Geometry: final body of the model. Coordinates: model frame, mm. A direction names the side the tool comes from. Round coordinates to 2 decimals unless told otherwise and drop trailing zeros. Write each loop counter-clockwise with the first axis right and the second up, starting at its lowest first coordinate (ties: lowest second). Pieces come first, ordered by that corner, then holes.
from build123d import *

# Parameters (mm, degrees)
F0_W      = 50.8
F0_H      = 457.2
F1_DEPTH  = 50.8
F2_R      = 4.699
F3_DEPTH  = 50.801
F5_DEPTH  = 50.801
F7_R      = 21.0312
F8_DEPTH  = 12.7
F9_R      = 16.002
F10_DEPTH = 12.7
F11_R     = 16.002
F12_DEPTH = 12.7
F13_R     = 3.175
F14_DEPTH = 12.7
F6_R      = 21.0312
F15_DEPTH = 12.7
F16_DEPTH = 12.7


with BuildPart() as f1:
    # F0 (on Front) → F1 (new body)
    with BuildSketch(Plane.XZ):
        Rectangle(F0_W, F0_H)
    extrude(amount=F1_DEPTH)

    # F2 (on face) → F3 (cut, through all)
    with BuildSketch(Plane.XZ.offset(50.8)):
        with Locations((0, -171.45)):
            Circle(F2_R)
        with Locations((0, -209.55)):
            Circle(F2_R)
    extrude(amount=-F3_DEPTH, mode=Mode.SUBTRACT)

    # F4 (on face) → F5 (cut, through all)
    with BuildSketch(Plane.XZ.offset(50.8)):
        with BuildLine():
            ThreePointArc((0, 173.43755), (14.310038, 179.364962), (20.23745, 193.675))
            ThreePointArc((20.23745, 193.675), (14.310038, 207.985038), (0, 213.91245))
            Line((0, 213.91245), (0, 193.675))
            Line((0, 193.675), (0, 173.43755))
        make_face()
        with BuildLine():
            ThreePointArc((15.20825, 152.4), (10.753857, 163.153857), (0, 167.60825))
            ThreePointArc((0, 167.60825), (-10.753857, 141.646143), (15.20825, 152.4))
        make_face()
        with BuildLine():
            Line((0, 193.675), (0, 213.91245))
            ThreePointArc((0, 213.91245), (-20.23745, 193.675), (0, 173.43755))
            Line((0, 173.43755), (0, 193.675))
        make_face()
    extrude(amount=-F5_DEPTH, mode=Mode.SUBTRACT)

    # F7 (on face) → F8 (cut)
    with BuildSketch(Plane(origin=(0, 0, 0), x_dir=(-1, 0, 0), z_dir=(0, 1, 0))):
        with Locations((0, 193.675)):
            Circle(F7_R)
    extrude(amount=-F8_DEPTH, mode=Mode.SUBTRACT)

    # F9 (on face) → F10 (cut)
    with BuildSketch(Plane.XZ.offset(50.8)):
        with Locations((0, 152.4)):
            Circle(F9_R)
    extrude(amount=-F10_DEPTH, mode=Mode.SUBTRACT)

    # F11 (on face) → F12 (cut)
    with BuildSketch(Plane(origin=(0, 0, 0), x_dir=(-1, 0, 0), z_dir=(0, 1, 0))):
        with Locations((0, 152.4)):
            Circle(F11_R)
    extrude(amount=-F12_DEPTH, mode=Mode.SUBTRACT)

    # F13 (on face) → F14 (cut)
    with BuildSketch(Plane.XZ.offset(50.8)):
        with Locations((15.478125, 170.32224)):
            Circle(F13_R)
        with Locations((0, 76.201982)):
            Circle(F13_R)
    extrude(amount=-F14_DEPTH, mode=Mode.SUBTRACT)

    # F6 (on face) → F15 (cut)
    with BuildSketch(Plane.XZ.offset(50.8)):
        with Locations((0, 193.675)):
            Circle(F6_R)
    extrude(amount=-F15_DEPTH, mode=Mode.SUBTRACT)

    # F6 (on face) → F16 (cut)
    with BuildSketch(Plane.XZ.offset(50.8)):
        with Locations((0, 193.675)):
            Circle(F6_R)
    extrude(amount=-F16_DEPTH, mode=Mode.SUBTRACT)


solid = f1.part
1) Section B-B on x = -10.5. Output: boundary loops of the cut face in (y, z).
2) Draft query along Z for faces 1 (the flat face through (0, -25, 228.6)), 2 (the cylindrical face through (3.47, -6.26, 136.78)), 3 (the flat face through (25.4, -25, -3)). Return one class per face: pulls with the +Z half, pulls with the -Z half, needs draft (parallel to the pull), parting line crosses it, or undercut.
3) Line query: probe 1 along Z at (x, y) = (0, -42.5); probe 2 along Z at (x, y) = (0, -8.25); probe 3 along X at (y, z) = (-25, -171). Output: solid intervals per line, ascending.
4) First-contact query: P1, Ø25, axis at x = 0, z = 193.675, coming from the +Y side; P2, Ø1.9, axis at x = 16.5, z = 169, coming from the -Y side. Flat tips, straight axial feed; report the tip coordinate or a pass-through.
5) Section A-A on z = -209.55. Output: boundary loops of the cut face in (x, y).
6) Section C-C on y = -46.5. Output: boundary loops of the cut face in (x, z) (3 decimals), plus the area to 3 significant figures.
7) Reachability of faces 4 (the flat face through (11, -12.7, 211)), 5 (the cylindrical face through (-3.47, -44.54, 136.78)), 6 (the flat face through (-25.4, -25, -3)) from +Z, -Z, +X, -X, +Y, -Y: full face, straight path, thin tool, end or side. Return the list, or none.
Filled in:
1. outline: (-50.8, -228.6) - (0, -228.6) - (0, 140.32) - (-12.7, 140.32) - (-12.7, 141.4) - (-38.1, 141.4) - (-38.1, 140.32) - (-50.8, 140.32) - close; (-50.8, 164.48) - (-38.1, 164.48) - (-38.1, 163.4) - (-12.7, 163.4) - (-12.7, 164.48) - (0, 164.48) - (0, 175.45) - (-12.7, 175.45) - (-12.7, 176.37) - (-38.1, 176.37) - (-38.1, 175.45) - (-50.8, 175.45) - close; (-50.8, 211.9) - (-38.1, 211.9) - (-38.1, 210.98) - (-12.7, 210.98) - (-12.7, 211.9) - (0, 211.9) - (0, 228.6) - (-50.8, 228.6) - close
2. face 1: pulls with the +Z half
2. face 2: undercut
2. face 3: needs draft
3. probe 1: z = -228.6 to -214.25, -204.85 to -176.15, -166.75 to 73.03, 79.38 to 136.4, 168.4 to 172.64, 214.71 to 228.6
3. probe 2: z = -228.6 to -214.25, -204.85 to -176.15, -166.75 to 136.4, 168.4 to 172.64, 214.71 to 228.6
3. probe 3: x = -25.4 to -4.68, 4.68 to 25.4
4. P1: passes through
4. P2: stops at y = -38.1
5. outline: (-25.4, -50.8) - (-4.7, -50.8) - (-4.7, 0) - (-25.4, 0) - close; (4.7, -50.8) - (25.4, -50.8) - (25.4, 0) - (4.7, 0) - close
6. outline: (-25.4, -228.6) - (25.4, -228.6) - (25.4, 228.6) - (-25.4, 228.6) - close; hole circle Ø42.062 at (0, 193.675); hole circle Ø32.004 at (0, 152.4); hole circle Ø9.398 at (0, -209.55); hole circle Ø9.398 at (0, -171.45); hole circle Ø6.35 at (0, 76.202); hole circle Ø6.35 at (15.478, 170.322)
6. area: 20,800 mm2
7. face 4: +Y
7. face 5: -Y
7. face 6: +Z, -Z, -X, +Y, -Y
